Source: CAD feature listing. Evaluate the final solid. Frame: model axes, mm. Round coordinates to 2 decimals unless told otherwise and drop trailing zeros. Loops run counter-clockwise (first coordinate to the right, second up) from the corner with the lowest first, then second, coordinate; pieces in that order, holes last. Notation, with made-up numbers: (58.5, 65) -> (78.5, 65) arc R19 ccw to (78.5, 79) -> close; hole circle Ø7 at (65.25, -9.5). An arc over 180 degrees is marked (long way). Write item = value, one per line.
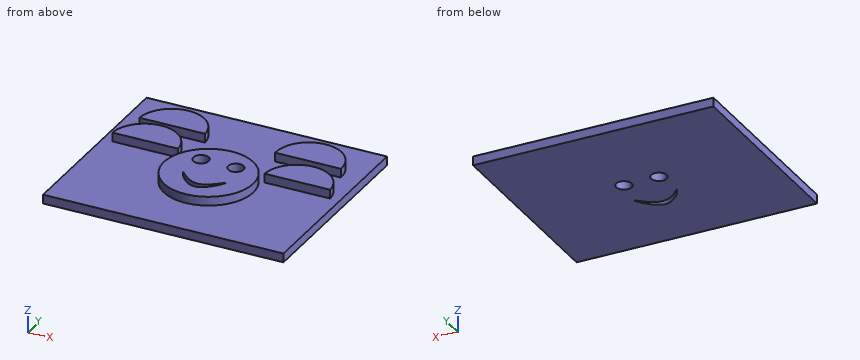
from build123d import *

# Parameters (mm, degrees)
F0_W     = 136.8003189564
F0_H     = 115.2591593564
F0_R     = 25.413882958
F1_DEPTH = 5.08
F2_DEPTH = 10.16
F0_R_2   = 4.445
F3_DEPTH = 10.16


# Not quite as in the source:
# - the program builds the solid bodies; features that only make, move or delete a surface that nothing else refers to are left out


with BuildPart() as f1:
    # F0 (on Top) → F1 (new body)
    with BuildSketch(Plane.XY):
        with Locations((0, 7.1337576956)):
            Rectangle(F0_W, F0_H)
        Circle(F0_R, mode=Mode.SUBTRACT)
        with BuildLine():
            Line((-25.4373313075, 15.699069947), (-62.7512871141, 15.699069947))
            ThreePointArc((-62.7512871141, 15.699069947), (-44.0943092108, 33.5629857305), (-25.4373313075, 15.699069947))
        make_face(mode=Mode.SUBTRACT)
        with BuildLine():
            Line((-20.3688811746, 35.9205551982), (-57.6828369811, 35.9205551982))
            ThreePointArc((-57.6828369811, 35.9205551982), (-39.0258590779, 53.7844709817), (-20.3688811746, 35.9205551982))
        make_face(mode=Mode.SUBTRACT)
        with BuildLine():
            Line((62.9981844539, 12.06225143), (25.6842286473, 12.06225143))
            ThreePointArc((25.6842286473, 12.06225143), (44.3412065506, 29.9261672135), (62.9981844539, 12.06225143))
        make_face(mode=Mode.SUBTRACT)
        with BuildLine():
            ThreePointArc((20.3699840242, 34.2742279379), (39.0258590779, 53.7844709817), (57.6817341315, 34.2742279379))
            Line((57.6817341315, 34.2742279379), (20.3699840242, 34.2742279379))
        make_face(mode=Mode.SUBTRACT)
    extrude(amount=F1_DEPTH)

    # F0 (on Top) → F2 (join)
    with BuildSketch(Plane.XY):
        with BuildLine():
            ThreePointArc((-20.3688811746, 35.9205551982), (-39.0258590779, 53.7844709817), (-57.6828369811, 35.9205551982))
            Line((-57.6828369811, 35.9205551982), (-20.3688811746, 35.9205551982))
        make_face()
        with BuildLine():
            ThreePointArc((-25.4373313075, 15.699069947), (-44.0943092108, 33.5629857305), (-62.7512871141, 15.699069947))
            Line((-62.7512871141, 15.699069947), (-25.4373313075, 15.699069947))
        make_face()
        with BuildLine():
            Line((20.3699840242, 34.2742279379), (57.6817341315, 34.2742279379))
            ThreePointArc((57.6817341315, 34.2742279379), (39.0258590779, 53.7844709817), (20.3699840242, 34.2742279379))
        make_face()
        with BuildLine():
            ThreePointArc((62.9981844539, 12.06225143), (44.3412065506, 29.9261672135), (25.6842286473, 12.06225143))
            Line((25.6842286473, 12.06225143), (62.9981844539, 12.06225143))
        make_face()
    extrude(amount=F2_DEPTH)

    # F0 (on Top) → F3 (join)
    with BuildSketch(Plane.XY):
        Circle(F0_R)
        with BuildLine():
            add(Edge.make_bspline(
                [(-11.889597401, -5.1754722372), (-11.6308932935, -4.6629733601), (-0.1804625636, -20.6748608417), (19.2699362073, 3.5560661133), (-0.2450377996, -26.2958289114), (-12.1664951894, -5.7240132208), (-11.889597401, -5.1754722372)],
                knots=[0, 0, 0, 0, 0.2394881843, 0.4838109378, 0.743669518, 1, 1, 1, 1], degree=3))
        make_face(mode=Mode.SUBTRACT)
        with Locations((-9.9313119426, 11.0503323376)):
            Circle(F0_R_2, mode=Mode.SUBTRACT)
        with Locations((9.9313119426, 11.0503323376)):
            Circle(F0_R_2, mode=Mode.SUBTRACT)
    extrude(amount=F3_DEPTH)


solid = f1.part
1. Section query C-C (y = -32). Return the cut outline in (x, z).
Evaluation:
outline = (-68.4, 0) -> (68.4, 0) -> (68.4, 5.08) -> (-68.4, 5.08) -> close
2. Section query B-B (x = 23.5). Return the cut outline in (y, z).
Evaluation:
outline = (-50.5, 0) -> (64.76, 0) -> (64.76, 5.08) -> (45.49, 5.08) -> (45.49, 10.16) -> (34.27, 10.16) -> (34.27, 5.08) -> (9.68, 5.08) -> (9.68, 10.16) -> (-9.68, 10.16) -> (-9.68, 5.08) -> (-50.5, 5.08) -> close
3. Section query A-A (y = 0). Return the cut outline in (x, z).
Evaluation:
outline = (-68.4, 0) -> (68.4, 0) -> (68.4, 5.08) -> (25.41, 5.08) -> (25.41, 10.16) -> (-25.41, 10.16) -> (-25.41, 5.08) -> (-68.4, 5.08) -> close
4. Line query: probe 1 along Z at (x, y) = (42, 32.5); probe 2 along Y at (x, z) = (-11, 4.75); probe 3 along Y at (x, z) = (-42, 8.5). Output: solid intervals per line, ascending. Write a range as from..to.
Evaluation:
probe_1 = 0..5.08
probe_2 = -50.5..-7.14, -5.88..6.74, 15.36..64.76
probe_3 = 15.7..33.45, 35.92..53.55
5. Contact query for flat-ended pins moving along their axis: pin 1 Ø1 at (x, z) = (-54.5, 5.5) entering from +Y; pin 2 Ø2.5 at (x, z) = (37, 8) entering from -Y; pin 3 Ø8 at (x, y) = (-9.93, 11.05) entering from +Z; pin 4 Ø2.5 at (x, z) = (-45, 6.5) entering from -Y. Output: stop coordinate, or through.
Evaluation:
pin_1 = 64.76
pin_2 = 12.06
pin_3 = through
pin_4 = 15.7
6. Section query D-D (x = -48). Return the cut outline in (y, z).
Evaluation:
outline = (-50.5, 0) -> (64.76, 0) -> (64.76, 5.08) -> (51.49, 5.08) -> (51.49, 10.16) -> (35.92, 10.16) -> (35.92, 5.08) -> (33.15, 5.08) -> (33.15, 10.16) -> (15.7, 10.16) -> (15.7, 5.08) -> (-50.5, 5.08) -> close
